Design review of the part built by this model. Coordinates are the model's own, in mm. Coordinates: 2 decimals unless noted, no trailing zeros. Order: outer loops, then holes, each group sorted by start corner. A loop starts at its lowest first (then second) coordinate and runs counter-clockwise, first axis right, second up. Notation, with made-up numbers: M 64,-1 L 110,-1 A33 cw 110,36 Z; hole C 46,44.25 d11. An arc over 180 degrees is marked long. Use CSV: the item, a comma, the result in double quotes.
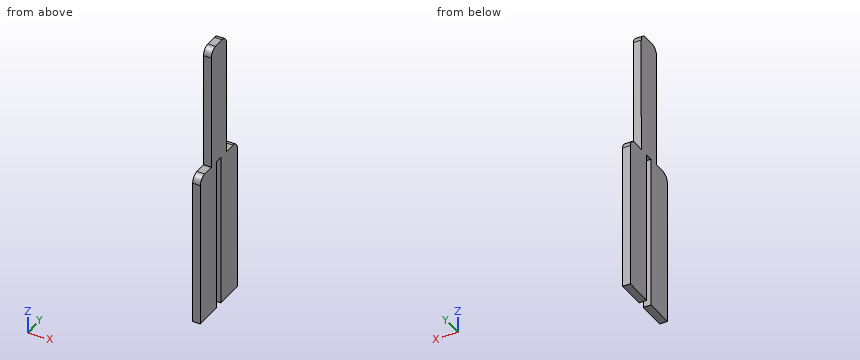
```python
from build123d import *

# Parameters (mm, degrees)
F1_DEPTH = 3.175


with BuildPart() as f1:
    # F0 (on Right) → F1 (new body, symmetric)
    with BuildSketch(Plane.YZ):
        with BuildLine():
            Line((3.175, -63.5), (26.9875, -63.5))
            Line((26.9875, -63.5), (26.9875, 57.15))
            ThreePointArc((26.9875, 57.15), (25.127628, 61.640128), (20.6375, 63.5))
            Line((20.6375, 63.5), (17.464617, 63.5))
            Line((17.464617, 63.5), (11.113911, 63.5))
            Line((11.113911, 63.5), (11.124494, 158.749293))
            ThreePointArc((11.124494, 158.749293), (9.264872, 163.239877), (4.774494, 165.099999))
            Line((4.774494, 165.099999), (-4.7498, 165.099999))
            ThreePointArc((-4.7498, 165.099999), (-9.239928, 163.240127), (-11.0998, 158.749999))
            Line((-11.0998, 158.749999), (-11.0998, 63.5))
            Line((-11.0998, 63.5), (-17.4498, 63.5))
            Line((-17.4498, 63.5), (-20.6375, 63.5))
            ThreePointArc((-20.6375, 63.5), (-25.127628, 61.640128), (-26.9875, 57.15))
            Line((-26.9875, 57.15), (-26.9875, -63.5))
            Line((-26.9875, -63.5), (-3.175, -63.5))
            Line((-3.175, -63.5), (-3.175, 63.5))
            Line((-3.175, 63.5), (3.175, 63.5))
            Line((3.175, 63.5), (3.175, -63.5))
        make_face()
    extrude(amount=F1_DEPTH, both=True)


solid = f1.part
```
(1) Add section A-A on z = 34. State the section outline as (x, y) points (1 decimal).
The answers:
outline,"M -3.2,-27 L 3.2,-27 L 3.2,-3.2 L -3.2,-3.2 Z; M -3.2,3.2 L 3.2,3.2 L 3.2,27 L -3.2,27 Z"
(2) Wall thickness on probe 1 along Y at (x, z) = (1, -48.5) (1 decimal); probe 2 along Z at (x, y) = (-2.5, 12); probe 3 along Y at (x, z) = (0.5, 77.5): over which ranges is each line inside the solid? List them lowest first.
The answers:
probe 1,"y = -27 to -3.2, 3.2 to 27"
probe 2,"z = -63.5 to 63.5"
probe 3,"y = -11.1 to 11.12"
(3) Add section D-D on z = 107. State the section outline as (x, y) points (3 decimals).
The answers:
outline,"M -3.175,-11.1 L 3.175,-11.1 L 3.175,11.119 L -3.175,11.119 Z"
(4) Add section C-C on y = 15. State the section outline as (x, z) points (3 decimals), and give its area (3 significant figures).
The answers:
outline,"M -3.175,-63.5 L 3.175,-63.5 L 3.175,63.5 L -3.175,63.5 Z"
area,"806 mm2"
(5) Clearance check with flat-ended pins moving along their axes: P1, Ø1.9, axis at x = 0, y = 1, coming from the -Z side; P2, Ø1.9, axis at x = 0.5, z = 94.5, coming from the +Y side; P3, Ø3, axis at x = -1.5, z = 97, coming from the -Y side. State where each tip first meets the part, or that it passes through.
The answers:
P1,"stops at z = 63.5"
P2,"stops at y = 11.12"
P3,"stops at y = -11.1"
